Source: CAD feature listing. Evaluate the final solid. Frame: model axes, mm. Face numbers are marked on the shaded views. A direction names the side the tool comes from. Give positions to 0.01 mm unless a question says otherwise; leave off trailing zeros. Loops run counter-clockwise (first coordinate to the right, second up) from the corner with the lowest first, then second, coordinate; pieces in that order, holes last. Notation, with made-up numbers: M 27.5,25.5 L 66.5,25.5 A14 cw 66.5,38.5 Z; hole C 81.25,82 d11. An arc over 180 degrees is marked long. Put each result on its own line as item: value.
from build123d import *

# Parameters (mm, degrees)
F1_DEPTH = 16.65056
F2_W     = 42
F2_H     = 42
F3_DEPTH = 2
F2_W_2   = 44
F2_H_2   = 44
F4_DEPTH = 15
F6_D     = 2.5
F7_DEPTH = 5.88
F8_W     = 1
F8_H     = 13.8298794627
F9_DEPTH = 25


with BuildPart() as f1:
    # F0 (on Top) → F1 (new body)
    with BuildSketch(Plane.XY):
        with BuildLine():
            Line((0.0728459244, 3.5), (4.8733971724, 3.5))
            ThreePointArc((4.8733971724, 3.5), (-6, 0), (4.8733971724, -3.5))
            Line((4.8733971724, -3.5), (0.0728459244, -3.5))
            Line((0.0728459244, -3.5), (0.0728459244, 3.5))
        make_face()
        with BuildLine():
            ThreePointArc((4.8733971724, 3.5), (5.7114088907, 1.8384255445), (6, 0))
            ThreePointArc((6, 0), (5.7114088907, -1.8384255445), (4.8733971724, -3.5))
            Line((4.8733971724, -3.5), (9.7837838487, -3.5))
            ThreePointArc((9.7837838487, -3.5), (8.6571810211, 0), (9.7837838487, 3.5))
            Line((9.7837838487, 3.5), (4.8733971724, 3.5))
        make_face()
        with BuildLine():
            ThreePointArc((4.8733971724, -3.5), (5.7114088907, -1.8384255445), (6, 0))
            ThreePointArc((6, 0), (5.7114088907, 1.8384255445), (4.8733971724, 3.5))
            Line((4.8733971724, 3.5), (0.0728459244, 3.5))
            Line((0.0728459244, 3.5), (0.0728459244, -3.5))
            Line((0.0728459244, -3.5), (4.8733971724, -3.5))
        make_face()
        with BuildLine():
            Line((14.6571810211, 3.5), (9.7837838487, 3.5))
            ThreePointArc((9.7837838487, 3.5), (8.6571810211, 0), (9.7837838487, -3.5))
            Line((9.7837838487, -3.5), (14.6571810211, -3.5))
            Line((14.6571810211, -3.5), (14.6571810211, 3.5))
        make_face()
        with BuildLine():
            ThreePointArc((20.6571810211, 0), (16.4956065656, 5.7114088907), (9.7837838487, 3.5))
            Line((9.7837838487, 3.5), (14.6571810211, 3.5))
            Line((14.6571810211, 3.5), (14.6571810211, -3.5))
            Line((14.6571810211, -3.5), (9.7837838487, -3.5))
            ThreePointArc((9.7837838487, -3.5), (16.4956065656, -5.7114088907), (20.6571810211, 0))
        make_face()
    extrude(amount=F1_DEPTH)

    # F2 (on face) → F3 (join)
    with BuildSketch(Plane.XY.offset(16.65056)):
        with Locations((7.3285905105, 0)):
            Rectangle(F2_W, F2_H)
        with BuildLine():
            ThreePointArc((4.8733971724, -3.5), (-6, 0), (4.8733971724, 3.5))
            Line((4.8733971724, 3.5), (9.7837838487, 3.5))
            ThreePointArc((9.7837838487, 3.5), (20.6571810211, 0), (9.7837838487, -3.5))
            Line((9.7837838487, -3.5), (4.8733971724, -3.5))
        make_face(mode=Mode.SUBTRACT)
        with BuildLine():
            Line((9.7837838487, 3.5), (4.8733971724, 3.5))
            ThreePointArc((4.8733971724, 3.5), (-6, 0), (4.8733971724, -3.5))
            Line((4.8733971724, -3.5), (9.7837838487, -3.5))
            ThreePointArc((9.7837838487, -3.5), (20.6571810211, 0), (9.7837838487, 3.5))
        make_face()
    extrude(amount=F3_DEPTH)

    # F2 (on face) → F4 (join)
    with BuildSketch(Plane.XY.offset(16.65056)):
        with Locations((7.3285905105, 0)):
            Rectangle(F2_W_2, F2_H_2)
        with Locations((7.3285905105, 0)):
            Rectangle(F2_W, F2_H, mode=Mode.SUBTRACT)
    extrude(amount=F4_DEPTH)

    # F6 (through all)
    with Locations(Plane(origin=(0, 0, 0), x_dir=(1, 0, 0), z_dir=(0, 0, -1))):
        with Locations((0, 0), (14.6571810211, 0)):
            Hole(F6_D / 2)

    # F7 (cut): a face of the model
    f7_faces = [f1.faces().sort_by_distance(p)[0] for p in [
        (7.3285905105, 0, 0),
    ]]
    extrude(f7_faces, amount=-F7_DEPTH, mode=Mode.SUBTRACT)

    # F8 (on face) → F9 (cut)
    with BuildSketch(Plane.XY.offset(31.65056)):
        with Locations((28.8285905105, 0.4071192816)):
            Rectangle(F8_W, F8_H)
    extrude(amount=-F9_DEPTH, mode=Mode.SUBTRACT)


solid = f1.part
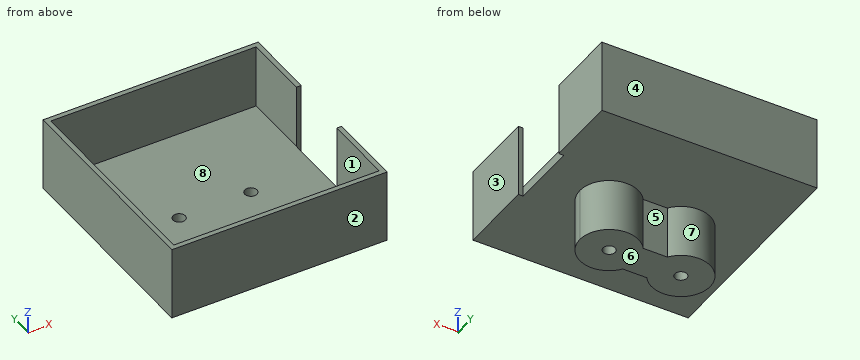
1. Material intervals for line 1 (Y direction, x = 0, z = 11.25); line 2 (Y direction, x = 14.5, z = 28.5); line 3 (X direction, y = -8, z = 19.5), sorted ascending. Write a range as from..to.
Found:
line 1: -6..-1.25, 1.25..6
line 2: -22..-21, 21..22
line 3: -14.67..-13.67, 28.33..29.33
2. Access query for the marked faces 4, 5, 6, 7 and 8. Directions: +Z, -Z, +X, -X, +Y, -Y. A direction counts if a zero-diameter tool reaches every point of the face in a straight line with its end or side. Return the directions, or none.
Found:
face 4: +Z, -Z, +X, -X, +Y
face 5: -Z, +Y
face 6: -Z, +X, -X, +Y, -Y
face 7: -Z
face 8: +Z
3. Section query B-B (z = 16). Output: boundary loops of the cut face in (x, y).
Found:
outline: M 4.87,-3.5 L 9.78,-3.5 A6 ccw long 9.78,3.5 L 4.87,3.5 A6 ccw long Z; hole C 0,0 d2.5; hole C 14.66,0 d2.5
4. Section query A-A (x = 0). Output: boundary loops of the cut face in (y, z).
Found:
outline: M -22,16.65 L -6,16.65 L -6,5.88 L -1.25,5.88 L -1.25,18.65 L -21,18.65 L -21,31.65 L -22,31.65 Z; M 1.25,5.88 L 6,5.88 L 6,16.65 L 22,16.65 L 22,31.65 L 21,31.65 L 21,18.65 L 1.25,18.65 Z
5. Draft query along Y for the marked faces 1, 2 and 3. Return one class per face: pulls with the +Y half, pulls with the -Y half, needs draft (parallel to the pull), parting line crosses it, or undercut.
Found:
face 1: undercut
face 2: pulls with the -Y half
face 3: needs draft
6. Contact query for flat-ended pins moving along their axis: P1, Ø1.5, axis at x = 0, y = 0, coming from the -Z side; P2, Ø4, axis at y = -3.5, z = 22, coming from the +X side; P3, Ø21, axis at x = 6, y = 7, coming from the +Z side; P4, Ø2.5, axis at x = 6.5, z = 11, coming from the +Y side. Output: stop coordinate, or through.
Found:
P1: through
P2: x = -13.67
P3: z = 18.65
P4: y = 3.5
7. Section query D-D (y = 2). Output: boundary loops of the cut face in (x, z), plus the area to 3 significant figures.
Found:
outline: M -14.67,16.65 L -5.66,16.65 L -5.66,5.88 L 20.31,5.88 L 20.31,16.65 L 28.33,16.65 L 28.33,18.65 L -13.67,18.65 L -13.67,31.65 L -14.67,31.65 Z
area: 379 mm^2
8. Section query C-C (x = -10.5). Output: boundary loops of the cut face in (y, z), plus the area to 3 significant figures.
Found:
outline: M -22,16.65 L 22,16.65 L 22,31.65 L 21,31.65 L 21,18.65 L -21,18.65 L -21,31.65 L -22,31.65 Z
area: 114 mm^2
